```python
from build123d import *

# Parameters (mm, degrees)
SKETCH1_W                     = 1209.675
SKETCH1_H                     = 72.3138
BASE_FLANGE1_DEPTH            = 3.175
EDGE_FLANGE1_STRIP_W          = 20.32
EDGE_FLANGE1_STRIP_H          = 3.175
EDGE_FLANGE1_STRIP_CUT_DEPTH  = 1209.675
EDGE_FLANGE1_DEPTH            = 1209.675
SKETCH10_W                    = 4.191
SKETCH10_H                    = 22.225
CUT_EXTRUDE2_DEPTH            = 611.335397201
FILLET1_R                     = 3.175
LPATTERN1_COUNT               = 2
LPATTERN1_PITCH               = 876.173
EDGE_FLANGE2_STRIP_W          = 20.32
EDGE_FLANGE2_STRIP_H          = 3.175
EDGE_FLANGE2_STRIP_CUT_DEPTH  = 50.8
EDGE_FLANGE2_RELIEF_W         = 21.9075
EDGE_FLANGE2_RELIEF_H         = 1.5875
EDGE_FLANGE2_RELIEF_CUT_DEPTH = 3.175
EDGE_FLANGE2_DEPTH            = 50.8
FILLET2_R                     = 3.175
F_10_0_1935_DIAMETER_HOLE1_D  = 4.9149


# Sheet-metal steps are written as plain solids
with BuildPart() as part:
    # Sketch1 → Base-Flange1 (new body)
    with BuildSketch(Plane(origin=(0, 0, 0), x_dir=(1, 0, 0), z_dir=(0, 1, 0))):
        with Locations((0, -36.1569)):
            Rectangle(SKETCH1_W, SKETCH1_H)
    extrude(amount=BASE_FLANGE1_DEPTH)

    # Edge-Flange1 strip (across the edge) → Edge-Flange1 strip cut (cut)
    with BuildSketch(Plane(origin=(604.8375, 3.175, 0), x_dir=(0, 0, 1), z_dir=(-1, 0, 0))):
        with Locations((-3.175, -1.5875)):
            Rectangle(EDGE_FLANGE1_STRIP_W, EDGE_FLANGE1_STRIP_H)
    extrude(amount=EDGE_FLANGE1_STRIP_CUT_DEPTH, mode=Mode.SUBTRACT)

    # Edge-Flange1 section (across the edge) → Edge-Flange1 (add)
    with BuildSketch(Plane(origin=(604.8375, 3.175, 0), x_dir=(0, 0, 1), z_dir=(-1, 0, 0))):
        with BuildLine():
            Line((0, 3.81), (0, 34.925))
            Line((0, 34.925), (3.175, 34.925))
            Line((3.175, 34.925), (3.175, 3.81))
            ThreePointArc((3.175, 3.81), (4.290923164, 1.115923164), (6.985, 0))
            Line((6.985, 0), (6.985, -3.175))
            ThreePointArc((6.985, -3.175), (2.045859133, -1.129140867), (0, 3.81))
        make_face()
    extrude(amount=EDGE_FLANGE1_DEPTH)

    # Sketch10 → Cut-Extrude2 (cut, through all)
    with BuildSketch(Plane(origin=(0, 0, 0), x_dir=(-1, 0, 0), z_dir=(0, 0, -1))):
        with Locations((433.324, 22.225)):
            Rectangle(SKETCH10_W, SKETCH10_H)
    cut_extrude2 = extrude(amount=-CUT_EXTRUDE2_DEPTH, mode=Mode.SUBTRACT)

    # Fillet1
    fillet1_edges = [part.edges().sort_by_distance(p)[0] for p in [
        (604.8375, 38.1, 1.5875),
        (-604.8375, 38.1, 1.5875),
        (-604.8375, 1.5875, 72.3138),
    ]]
    fillet(fillet1_edges, radius=FILLET1_R)

    # LPattern1: Cut-Extrude2 ×2
    with Locations(*[(i * LPATTERN1_PITCH, 0, 0) for i in range(1, LPATTERN1_COUNT)]):
        add(cut_extrude2, mode=Mode.SUBTRACT)

    # Edge-Flange2 strip (across the edge) → Edge-Flange2 strip cut (cut)
    with BuildSketch(Plane(origin=(554.0375, 3.175, 72.3138), x_dir=(0, 0, -1), z_dir=(1, 0, 0))):
        with Locations((-6.35, -1.5875)):
            Rectangle(EDGE_FLANGE2_STRIP_W, EDGE_FLANGE2_STRIP_H)
    extrude(amount=EDGE_FLANGE2_STRIP_CUT_DEPTH, mode=Mode.SUBTRACT)

    # Edge-Flange2 relief (on the sheet) → Edge-Flange2 relief cut (cut)
    with BuildSketch(Plane(origin=(554.0375, 3.175, 68.5038), x_dir=(0, 0, -1), z_dir=(0, 1, 0))):
        with Locations((-9.36625, 0.79375)):
            Rectangle(EDGE_FLANGE2_RELIEF_W, EDGE_FLANGE2_RELIEF_H)
    extrude(amount=-EDGE_FLANGE2_RELIEF_CUT_DEPTH, mode=Mode.SUBTRACT)

    # Edge-Flange2 section (across the edge) → Edge-Flange2 (add)
    with BuildSketch(Plane(origin=(554.0375, 3.175, 72.3138), x_dir=(0, 0, -1), z_dir=(1, 0, 0))):
        with BuildLine():
            Line((-3.175, 3.81), (-3.175, 34.925))
            Line((-3.175, 34.925), (0, 34.925))
            Line((0, 34.925), (0, 3.81))
            ThreePointArc((0, 3.81), (1.115923164, 1.115923164), (3.81, 0))
            Line((3.81, 0), (3.81, -3.175))
            ThreePointArc((3.81, -3.175), (-1.129140867, -1.129140867), (-3.175, 3.81))
        make_face()
    extrude(amount=EDGE_FLANGE2_DEPTH)

    # Fillet2
    fillet2_edges = [part.edges().sort_by_distance(p)[0] for p in [
        (554.0375, 38.1, 73.9013),
        (604.8375, 38.1, 73.9013),
    ]]
    fillet(fillet2_edges, radius=FILLET2_R)

    # #10 (0.1935) Diameter Hole1 (through all)
    with Locations(Plane.XY.offset(75.4888)):
        with Locations((590.55, 19.05), (565.15, 19.05)):
            Hole(F_10_0_1935_DIAMETER_HOLE1_D / 2)


solid = part.part
```
Build history of the part. All positions in model axes, mm. Coordinates: 2 decimals unless noted, no trailing zeros. Write each loop counter-clockwise with the first axis right and the second up, starting at its lowest first coordinate (ties: lowest second). Pieces come first, ordered by that corner, then holes.
1. Pull direction Z, two halves, no side cores. Call faces 1 (the flat face through (-604.838, 2, 24)), 2 (the flat face through (8, 22, 0)), 3 (the flat face through (579, 23, 72.314)): released by +Z, released by -Z, zero draft, split by the parting line, or undercut.
Answer block:
face 1: zero draft
face 2: released by -Z
face 3: undercut
2. Drop flat-ended pins along their axis: pin 1 (1.6 mm diameter, centred on x = 88.5, y = 1, fed in from +Z); pin 2 (1.5 mm diameter, centred on x = 214, y = 26, fed in from +Z) (3 decimals); pin 3 (4 mm diameter, centred on x = 565.15, y = 19.05, fed in from -Z); pin 4 (3.5 mm diameter, centred on x = 442.5, z = 1, fed in from -Y). Give the stop position or say it passes through.
Answer block:
pin 1: stops at z = 72.31
pin 2: stops at z = 3.175
pin 3: passes through
pin 4: stops at y = 1.43
3. Band-saw the part on A-A, the plane x = 31. Give the cut face in (y, z) (3 decimals).
Answer block:
outline: (0, 6.985) arc R6.985 ccw to (6.985, 0) - (38.1, 0) - (38.1, 3.175) - (6.985, 3.175) arc R3.81 cw to (3.175, 6.985) - (3.175, 72.314) - (0, 72.314) - close
4. Band-saw the part on B-B, the plane z = 46.5. Give the cut face in (x, y) (1 decimal).
Answer block:
outline: (-604.8, 0) - (604.8, 0) - (604.8, 3.2) - (-604.8, 3.2) - close
5. Drill centre lines: probe 1 along X at (y, z) = (19, 2); probe 2 along X at (y, z) = (19, 73); probe 3 along Z at (x, y) = (-166.5, 21) (3 decimals). Where is each one in solid material? Low to high.
Answer block:
probe 1: x = -604.84 to -435.42, -431.23 to 440.75, 444.94 to 562.69, 567.61 to 588.09, 593.01 to 604.84
probe 2: x = 554.04 to 562.69, 567.61 to 588.09, 593.01 to 604.84
probe 3: z = 0 to 3.175
